Autodesk Inventor part; units mm, degrees
ref_plane "YZ Plane" through (0, 0, 0) normal (1, 0, 0) x (0, 1, 0)
ref_plane "XZ Plane" through (0, 0, 0) normal (0, 1, 0) x (-1, 0, 0)
ref_plane "XY Plane" through (0, 0, 0) normal (0, 0, 1) x (1, 0, 0)
sketch "スケッチ1" plane through (0, 0, 0) normal (0, 0, 1) x (1, 0, 0)
  circle A0 centre (0, 0) radius 42.5 construction
  arc A1 (71.9037, -6.5306) -> (71.9037, 6.5306) centre (53, 0) ccw
  circle A2 centre (53, 0) radius 49 construction
  arc A3 (-5.838, 3.8623) -> (-5.838, -3.8623) centre (0, 0) ccw
  arc A4 (19.4901, 40.7594) -> (17.317, 38.812) centre (20.8892, 37.0121) ccw
  arc A5 (17.317, -38.812) -> (19.4901, -40.7594) centre (20.8892, -37.0121) ccw
  arc A6 (56.7807, 50.3061) -> (51.601, 52.7474) centre (53, 49) ccw
  arc A7 (51.601, -52.7474) -> (56.7807, -50.3061) centre (53, -49) ccw
  line L0 (19.4901, 40.7594) -> (51.601, 52.7474)
  line L1 (56.7807, 50.3061) -> (71.9037, 6.5306)
  line L2 (71.9037, -6.5306) -> (56.7807, -50.3061)
  line L3 (51.601, -52.7474) -> (19.4901, -40.7594)
  line L4 (17.5531, -39.2191) -> (-5.838, -3.8623)
  line L5 (-5.838, 3.8623) -> (17.5531, 39.2191)
  dimension "d0" = 53
  dimension "d1" = 40
  dimension "d2" = 98
  dimension "d3" = 85
  dimension "d4" = 14
  dimension "d5" = 8
  dimension "d6" = 8
  dimension "d7" = 8
  dimension "d8" = 8
extrude "プレート1" add sketch "スケッチ1" along normal blind 2.3
sketch "スケッチ2" plane through (0, 0, 2.3) normal (0, 0, 1) x (1, 0, 0)
  arc A0 (71.9037, -6.5306) -> (71.9037, 6.5306) centre (53, 0) ccw
  line L0 (56.7807, 50.3061) -> (71.9037, 6.5306)
  arc A1 (56.7807, 50.3061) -> (51.601, 52.7474) centre (53, 49) ccw
  line L1 (19.4901, 40.7594) -> (51.601, 52.7474)
  arc A2 (19.4901, 40.7594) -> (17.5531, 39.2191) centre (20.8892, 37.0121) ccw
  line L2 (-5.838, 3.8623) -> (17.5531, 39.2191)
  arc A3 (-5.838, 3.8623) -> (-5.838, -3.8623) centre (0, 0) ccw
  line L3 (17.5531, -39.2191) -> (-5.838, -3.8623)
  arc A4 (17.5531, -39.2191) -> (19.4901, -40.7594) centre (20.8892, -37.0121) ccw
  line L4 (51.601, -52.7474) -> (19.4901, -40.7594)
  arc A5 (51.601, -52.7474) -> (56.7807, -50.3061) centre (53, -49) ccw
  line L5 (71.9037, -6.5306) -> (56.7807, -50.3061)
hole "穴1" at (53, 49, 2.3) at (53, -49, 2.3) at (20.8892, 37.0121, 2.3) at (20.8892, -37.0121, 2.3) direction (0, 0, -1) diameter 4.3 depth 2.3
sketch "スケッチ3" plane through (0, 0, 2.3) normal (0, 0, 1) x (1, 0, 0)
  arc A0 (71.9037, -6.5306) -> (71.9037, 6.5306) centre (53, 0) ccw
  circle A1 centre (53, 0) radius 10
  point P0 (0, 0)
  dimension "d17" = 20
extrude "押し出し1" cut sketch "スケッチ3" against normal blind 10
sketch "スケッチ4" plane through (0, 0, 2.3) normal (0, 0, 1) x (1, 0, 0)
  arc A0 (71.9037, -6.5306) -> (71.9037, 6.5306) centre (53, 0) ccw
  circle A1 centre (53, 0) radius 15
  point P0 (0, 0)
  point P1 (38, 0)
  point P2 (53, -15)
  point P3 (68, 0)
  point P4 (53, 15)
  dimension "d20" = 30
  dimension "d23" = 360
hole "穴2" at (38, 0, 2.3) at (53, -15, 2.3) at (68, 0, 2.3) at (53, 15, 2.3) direction (0, 0, -1) diameter 3.2 depth 2.3
sketch "スケッチ5" plane through (0, 0, 2.3) normal (0, 0, 1) x (1, 0, 0)
  arc A0 (71.9037, -6.5306) -> (71.9037, 6.5306) centre (53, 0) ccw
  circle A1 centre (53, 0) radius 16
  point P0 (0, 0)
  point P1 (41.6863, 11.3137)
  point P2 (41.6863, -11.3137)
  point P3 (64.3137, -11.3137)
  point P4 (64.3137, 11.3137)
  dimension "d32" = 32
  dimension "d35" = 360
hole "穴3" at (41.6863, 11.3137, 2.3) at (41.6863, -11.3137, 2.3) at (64.3137, -11.3137, 2.3) at (64.3137, 11.3137, 2.3) direction (0, 0, -1) diameter 4.3 depth 2.3
sketch "スケッチ6" plane through (0, 0, 2.3) normal (0, 0, 1) x (1, 0, 0)
  arc A0 (-5.838, 3.8623) -> (-5.838, -3.8623) centre (0, 0) ccw
hole "穴4" at (0, 0, 2.3) direction (0, 0, -1) diameter 4.3 depth 2.3
sketch "スケッチ7" plane through (0, 0, 2.3) normal (0, 0, 1) x (1, 0, 0)
  line L0 (-1.5, 0) -> (1.5, 0) construction
  line L1 (-1.5, -2.15) -> (1.5, -2.15)
  line L2 (1.5, 2.15) -> (-1.5, 2.15)
  arc A0 (-1.5, 2.15) -> (-1.5, -2.15) centre (-1.5, 0) ccw
  arc A1 (1.5, -2.15) -> (1.5, 2.15) centre (1.5, 0) ccw
  circle A2 centre (0, 0) radius 2.15
  point P0 (0, 2.15)
  point P1 (0, -2.15)
  dimension "d51" = 3
extrude "押し出し2" cut sketch "スケッチ7" against normal blind 10
equation "\"d15\" = Thickness"
equation "\"d30\" = Thickness"
equation "\"d42\" = Thickness"
equation "\"d49\" = Thickness"
equation "\"d9\" = Thickness"
equation "\"BendRadius\" = Thickness"
equation "\"BendReliefWidth\" = Thickness"
equation "\"BendReliefDepth\" = 0.5 * Thickness"
equation "\"CornerReliefSize\" = 4 * Thickness"
equation "\"MinimumRemnant\" = 2 * Thickness"
equation "\"TransitionRadius\" = BendRadius"
equation "\"JacobiRadiusSize\" = BendRadius"
equation "\"GapSize\" = Thickness"
properties part number "steel_plate7" material "鋼、炭素鋼"
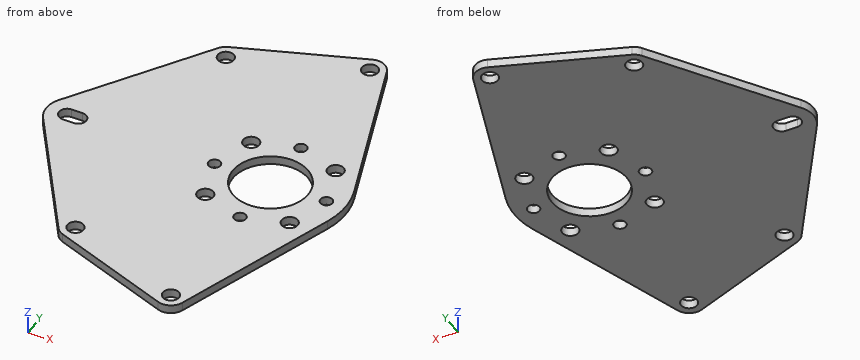
For this review, take the finished solid that the model builds, in its own axes (mm). Coordinates: 2 decimals unless noted, no trailing zeros. Write each loop counter-clockwise with the first axis right and the second up, starting at its lowest first coordinate (ties: lowest second). Pieces come first, ordered by that corner, then holes. Notation, with made-up numbers: (-2.75, 36) - (51.25, 36) arc R5 cw to (51.25, 43) - close; hole circle Ø8 at (8.5, 14.5). An arc over 180 degrees is marked (long way). Put each result on its own line as item: value.
1. Add section B-B, the plane y = 15. Give the boundary of the cut face in (x, z).
Values found:
outline: (1.53, 0) - (51.4, 0) - (51.4, 2.3) - (1.53, 2.3) - close; (54.6, 0) - (68.98, 0) - (68.98, 2.3) - (54.6, 2.3) - close
2. Add section A-A, the plane x = 53. Give the boundary of the cut face in (y, z), then the cut area to 3 significant figures.
Values found:
outline: (-53, 0) - (-51.15, 0) - (-51.15, 2.3) - (-53, 2.3) - close; (-46.85, 0) - (-16.6, 0) - (-16.6, 2.3) - (-46.85, 2.3) - close; (-13.4, 0) - (-10, 0) - (-10, 2.3) - (-13.4, 2.3) - close; (10, 0) - (13.4, 0) - (13.4, 2.3) - (10, 2.3) - close; (16.6, 0) - (46.85, 0) - (46.85, 2.3) - (16.6, 2.3) - close; (51.15, 0) - (53, 0) - (53, 2.3) - (51.15, 2.3) - close
area: 163 mm²
3. Add section C-C, the plane x = 38. Give the boundary of the cut face in (y, z), then the cut area to 3 significant figures.
Values found:
outline: (-47.67, 0) - (-1.6, 0) - (-1.6, 2.3) - (-47.67, 2.3) - close; (1.6, 0) - (47.67, 0) - (47.67, 2.3) - (1.6, 2.3) - close
area: 212 mm²
4. Wall thickness on probe 1 along Y at (x, z) = (53, 1); probe 2 along X at (y, z) = (-3, 1.7); probe 3 along X at (y, z) = (36, 1.3): over which ranges is each line inside the solid? List them lowest first.
Values found:
probe 1: -53 to -51.15, -46.85 to -16.6, -13.4 to -10, 10 to 13.4, 16.6 to 46.85, 51.15 to 53
probe 2: -6.32 to 43.46, 62.54 to 72.77
probe 3: 15.42 to 18.99, 22.79 to 61.72
5. Add section D-D, the plane z = 0.45. Count the separate pieces of the cut face and the enclosed holes in it, then the cut area to 3 significant figures.
Values found:
separate pieces: 1
enclosed holes: 14
area: 5,090 mm²
